Input: part model. Units: mm. Frame: model coordinates. A direction names the side the tool comes from. Coordinates: 2 decimals unless noted, no trailing zeros. Write each loop counter-clockwise with the first axis right and the second up, starting at its lowest first coordinate (ties: lowest second). Pieces come first, ordered by that corner, then holes.
Autodesk Inventor part; units mm, degrees
ref_plane "Arbeitsebene1" through (0, 0, 30) normal (0, 0, 1) x (1, 0, 0)
ref_plane "YZ Plane" through (0, 0, 0) normal (1, 0, 0) x (0, 1, 0)
ref_plane "XZ Plane" through (0, 0, 0) normal (0, 1, 0) x (-1, 0, 0)
sketch "Skizze1" plane through (0, 0, 0) normal (0, 0, 1) x (1, 0, 0)
  line L0 (-28, 0) -> (28, 0)
  line L1 (0, -28) -> (0, 28)
  circle A0 centre (0, 0) radius 20
  dimension "d0" = 40
extrude "Extrusion1" add sketch "Skizze1" along normal blind 15
sketch "Skizze2" plane through (0, 0, 15) normal (0, 0, 1) x (1, 0, 0)
  circle A0 centre (0, 0) radius 7.5
  dimension "d3" = 15
extrude "Extrusion2" add sketch "Skizze2" along normal blind 20
fillet "Rundung1" radius 5 1 edges at (-7.5, 0, 15)
chamfer "Fase1" distance 1 angle 45 2 edges at (-20, 0, 15) (-20, 0, 0)
fillet "Rundung2" radius 2 1 edges at (-7.5, 0, 35)
ref_plane "Arbeitsebene1" through (0, 0, 30) normal (0, 0, 1) x (1, 0, 0)
sketch "Skizze4" plane through (0, 0, 30) normal (0, 0, 1) x (1, 0, 0)
  circle A0 centre (0, 0) radius 5.5
  circle A1 centre (0, 0) radius 7.5
extrude "Extrusion3" cut sketch "Skizze4" along normal mid plane 1
fillet "Rundung3" radius 0.5 2 edges at (-7.5, 0, 30.5) (-7.5, 0, 29.5)
sketch "Skizze5" plane through (0, 0, 35) normal (0, 0, 1) x (1, 0, 0)
  circle A0 centre (0, 0) radius 4.5
  dimension "d15" = 9
extrude "Extrusion4" cut sketch "Skizze5" against normal blind 40
sketch "Skizze6" plane through (0, 0, 0) normal (0, 0, -1) x (-1, 0, 0)
  circle A0 centre (0, 0) radius 15
  dimension "d18" = 30
extrude "Extrusion5" cut sketch "Skizze6" against normal blind 12
thread "Gewinde1"
chamfer "Fase2" distance 1 angle 45 1 edges at (15, 0, 0)
chamfer "Fase3" distance 1 angle 45 1 edges at (-4.5, 0, 12)
properties part number "SchlauchAnschluss"
Item 1: Pull-direction query (X, two-part tool) for faces 1 (the face through (0, -6, 12)), 2 (the face through (-1.19, -5.37, 30.01)), 3 (the face through (-4, -4, 29.5)), 4 (the face through (-0.59, 4.46, 24.15)); classes: released by +X, released by -X, zero draft, split by the parting line, or undercut.
Item 2: Section query B-B, the plane z = 22.5. Return loops of the section in (x, y).
Item 3: Material intervals for line 1 (Y direction, x = 0, z = 3); line 2 (Y direction, x = 0, z = 27.75); line 3 (X direction, y = 5, z = 7), sorted ascending.
Item 4: Pin query (flat end, axial travel): pin 1 Ø7 at (x, y) = (0, 0) entering from +Z; pin 2 Ø11 at (x, y) = (-2, -2.5) entering from -Z; pin 3 Ø4 at (x, y) = (15, -6.5) entering from +Z; pin 4 Ø1.5 at (x, z) = (-0.5, 14.5) entering from -Y. Return the tip coordinate at first contact, or that it passes through.
Item 5: Section query A-A, the plane z = 9. Return loops of the section in (x, y).
Item 6: Access query for faces 5 (the face through (-4, -4, 30.5)), 6 (the face through (4, -12.4, 15)), 7 (the face through (14.985, 0.66, 6.423)). Directions: +Z, -Z, +X, -X, +Y, -Y. A direction counts if a zero-diameter tool reaches every point of the face in a straight line with its end or side. Return the directions, or none.
The answers:
1. face 1: undercut
1. face 2: split by the parting line
1. face 3: zero draft
1. face 4: undercut
2. outline: circle Ø15 at (0, 0); hole circle Ø9 at (0, 0)
3. line 1: y = -20 to -15, 15 to 20
3. line 2: y = -7.5 to -4.5, 4.5 to 7.5
3. line 3: x = -19.36 to -14.14, 14.14 to 19.36
4. pin 1: passes through
4. pin 2: stops at z = 12
4. pin 3: stops at z = 15
4. pin 4: stops at y = -20
5. outline: circle Ø40 at (0, 0); hole circle Ø30 at (0, 0)
6. face 5: none
6. face 6: +Z
6. face 7: -Z
